```python
from build123d import *

# Parameters (mm, degrees)
SKETCH1_W           = 326.39
SKETCH1_H           = 88.9
SKETCH1_W_2         = 300.99
SKETCH1_H_2         = 76.2
BOSS_EXTRUDE1_DEPTH = 50.8
SKETCH2_W           = 326.39
SKETCH2_H           = 88.9
BOSS_EXTRUDE2_DEPTH = 6.35
SKETCH3_R           = 3.1
CUT_EXTRUDE1_DEPTH  = 179.534402917
SKETCH4_R           = 1.6875
CUT_EXTRUDE3_DEPTH  = 313.69


with BuildPart() as part:
    # Sketch1 → Boss-Extrude1 (new body)
    with BuildSketch(Plane(origin=(0, 0, 0), x_dir=(1, 0, 0), z_dir=(0, 1, 0))):
        Rectangle(SKETCH1_W, SKETCH1_H)
        Rectangle(SKETCH1_W_2, SKETCH1_H_2, mode=Mode.SUBTRACT)
    extrude(amount=BOSS_EXTRUDE1_DEPTH)

    # Sketch2 → Boss-Extrude2 (add)
    with BuildSketch(Plane.XZ):
        Rectangle(SKETCH2_W, SKETCH2_H)
    extrude(amount=BOSS_EXTRUDE2_DEPTH)

    # Sketch3 → Cut-Extrude1 (cut, through all)
    with BuildSketch(Plane.XZ.offset(6.35)):
        with Locations(Location((-106, 7.5, 0), (0, 0, 270))):
            Circle(SKETCH3_R)
        with Locations(Location((-106, -7.5, 0), (0, 0, 270))):
            Circle(SKETCH3_R)
    extrude(amount=-CUT_EXTRUDE1_DEPTH, mode=Mode.SUBTRACT)

    # Sketch4 → Cut-Extrude3 (cut)
    with BuildSketch(Plane(origin=(163.195, 0, 0), x_dir=(0, 0, -1), z_dir=(1, 0, 0))):
        with Locations((25.4, 44.22394)):
            Circle(SKETCH4_R)
        with Locations(Location((-25.4, 44.22394, 0), (0, 0, 180))):
            Circle(SKETCH4_R)
    cut_extrude3 = extrude(amount=-CUT_EXTRUDE3_DEPTH, mode=Mode.SUBTRACT)

    # Mirror2: Cut-Extrude3 across plane
    add(cut_extrude3.mirror(Plane(origin=(0, 0, 0), x_dir=(0, 0, 1), z_dir=(1, 0, 0))), mode=Mode.SUBTRACT)


solid = part.part
```
Can you work these out from the model? Positions are in its coordinate system, mm. A direction names the side the tool comes from. Coordinates: 2 decimals unless noted, no trailing zeros. Loops run counter-clockwise (first coordinate to the right, second up) from the corner with the lowest first, then second, coordinate; pieces in that order, holes last.
Item 1: Which directions (+Z, -Z, +X, -X, +Y, -Y) give clear straight access to the entire face, cutting with the end or side of a thin tool? Please do faces 5 (the face through (-2, -6.35, 1)), 6 (the face through (150.495, 25, 1)).
Answers below:
face 5: +Z, -Z, +X, -X, -Y
face 6: +Y
Item 2: Suppose I cut it at C-C (y = 10). Please give me the cut outline in (x, z) (3 decimals), then the cut area to 3 significant figures.
Answers below:
outline: (-163.195, -44.45) - (163.195, -44.45) - (163.195, 44.45) - (-163.195, 44.45) - close; hole (-150.495, -38.1) - (150.495, -38.1) - (150.495, 38.1) - (-150.495, 38.1) - close
area: 6,080 mm2
Item 3: Suppose I cut it at D-D (z = -31). Please give me the cut outline in (x, y) (3 decimals), then the cut area to 3 significant figures.
Answers below:
outline: (-163.195, -6.35) - (163.195, -6.35) - (163.195, 50.8) - (150.495, 50.8) - (150.495, 0) - (-150.495, 0) - (-150.495, 50.8) - (-163.195, 50.8) - close
area: 3,360 mm2
Item 4: Please list where these lines run through material, in increasing order: L1, parallel to Z at x = -22.5, y = 23; L2, parallel to X at y = -3, z = 7 (3 decimals); L3, parallel to X at y = 41, z = 23 (3 decimals).
Answers below:
L1: z = -44.45 to -38.1, 38.1 to 44.45
L2: x = -163.195 to -109.059, -102.941 to 163.195
L3: x = -163.195 to -150.495, 150.495 to 163.195
Item 5: Suppose I cut it at B-B (z = -7.5). Please give me the cut outline in (x, y) (3 decimals), then the cut area to 3 significant figures.
Answers below:
outline: (-163.195, -6.35) - (-109.1, -6.35) - (-109.1, 0) - (-150.495, 0) - (-150.495, 50.8) - (-163.195, 50.8) - close; (-102.9, -6.35) - (163.195, -6.35) - (163.195, 50.8) - (150.495, 50.8) - (150.495, 0) - (-102.9, 0) - close
area: 3,320 mm2
Item 6: Suppose I cut it at A-A (x = -106). Please give me the cut outline in (y, z).
Answers below:
outline: (-6.35, -44.45) - (50.8, -44.45) - (50.8, -38.1) - (0, -38.1) - (0, -10.6) - (-6.35, -10.6) - close; (-6.35, -4.4) - (0, -4.4) - (0, 4.4) - (-6.35, 4.4) - close; (-6.35, 10.6) - (0, 10.6) - (0, 38.1) - (50.8, 38.1) - (50.8, 44.45) - (-6.35, 44.45) - close
Item 7: If we mould it in two halves opening along Z, with no side actions, what happens to faces 1 (the face through (-150.495, 25, 1)), 2 (the face through (-2, 23, 44.45)), 3 (the face through (-2, 0, 1)), 4 (the face through (-13, 50.8, 39))? For each: released by +Z, released by -Z, zero draft, split by the parting line, or undercut.
Answers below:
face 1: undercut
face 2: released by +Z
face 3: undercut
face 4: zero draft
Item 8: I'm going to push flat-ended pins straight in: pin 1 (2.5 mm diameter, centred on y = 44.22, z = -25.4, fed in from +X); pin 2 (10 mm diameter, centred on x = -106, z = 7.5, fed in from -Y). Where does each tip first touch, or does it pass through?
Answers below:
pin 1: passes through
pin 2: stops at y = -6.35
